The model under review builds one solid part; all positions refer to its coordinate system, in mm. Coordinates: 2 decimals unless noted, no trailing zeros. Write each loop counter-clockwise with the first axis right and the second up, starting at its lowest first coordinate (ties: lowest second). Pieces come first, ordered by that corner, then holes.
```python
from build123d import *

# Parameters (mm, degrees)
BOSS_EXTRUDE1_DEPTH  = 0.79375
M4_CLEARANCE_HOLE1_D = 4.8


with BuildPart() as part:
    # Sketch1 → Boss-Extrude1 (new, symmetric)
    with BuildSketch(Plane(origin=(0, 0, 0), x_dir=(0, 0, -1), z_dir=(1, 0, 0))):
        with BuildLine():
            Line((-5.08, 12.7), (-5.08, -6.538207725))
            ThreePointArc((-5.08, -6.538207725), (-5.211700121, -7.824771606), (-5.601337517, -9.057968362))
            Line((-5.601337517, -9.057968362), (-21.415741229, -45.63954689))
            ThreePointArc((-21.415741229, -45.63954689), (-7.844956242, -39.930269315), (2.000109042, -50.877266399))
            Line((2.000109042, -50.877266399), (5.062707082, -9.46401976))
            ThreePointArc((5.062707082, -9.46401976), (5.075675298, -9.230020736), (5.08, -8.995702545))
            Line((5.08, -8.995702545), (5.08, 12.7))
            ThreePointArc((5.08, 12.7), (0, 17.78), (-5.08, 12.7))
        make_face()
    extrude(amount=BOSS_EXTRUDE1_DEPTH, both=True)

    # M4 Clearance Hole1 (through all)
    with Locations(Plane(origin=(0.79375, 0, 0), x_dir=(0, 0, -1), z_dir=(1, 0, 0))):
        with Locations((0, 0), (0, 12.7), (0, -12.7)):
            Hole(M4_CLEARANCE_HOLE1_D / 2)


solid = part.part
```
Item 1: Take a section at D-D, the plane y = -12.7. Write out the cut boundary in (x, z).
Solved:
outline: (-0.79, -4.82) - (0.79, -4.82) - (0.79, -2.4) - (-0.79, -2.4) - close; (-0.79, 2.4) - (0.79, 2.4) - (0.79, 7.18) - (-0.79, 7.18) - close
Item 2: Mouldability with a two-part tool opening along Z and no side actions: class faces 1 (the face through (-0.794, -16, 2)), 2 (the face through (0, 3, 5.08)), 3 (the face through (0, 2, -5.08)), 4 (the face through (-0.011, 14.724, 1.29)) as pulls with the +Z half, pulls with the -Z half, needs draft (parallel to the pull), parting line crosses it, or undercut.
Solved:
face 1: needs draft
face 2: pulls with the +Z half
face 3: pulls with the -Z half
face 4: undercut
Item 3: For pin 1 (6 mm diameter, centred on y = -12.7, z = 0, fed in from -X); pin 2 (0.5 mm diameter, centred on x = 0, y = 6.5, fed in from +Z), all flat-tipped, find the tip position at first contact; note any pin that passes through.
Solved:
pin 1: stops at x = -0.79
pin 2: stops at z = 5.08
Item 4: Take a section at A-A, the plane x = 0.25. Write out the cut boundary in (y, z).
Solved:
outline: (-50.88, -2) - (-9.46, -5.06) arc R6.35 ccw to (-9, -5.08) - (12.7, -5.08) arc R5.08 ccw to (12.7, 5.08) - (-6.54, 5.08) arc R6.35 cw to (-9.06, 5.6) - (-45.64, 21.42) arc R12.7 cw to start; hole circle Ø4.8 at (-12.7, 0); hole circle Ø4.8 at (0, 0); hole circle Ø4.8 at (12.7, 0)
Item 5: Take a section at B-B, the plane y = 0. Write out the cut boundary in (x, z).
Solved:
outline: (-0.79, -5.08) - (0.79, -5.08) - (0.79, -2.4) - (-0.79, -2.4) - close; (-0.79, 2.4) - (0.79, 2.4) - (0.79, 5.08) - (-0.79, 5.08) - close
Item 6: To check wall thickness, follow line 1 along Y through (x, z) = (0.45, 0); line 2 along Z through (x, y) = (0.4, 6.5); line 3 along Y through (x, z) = (0.1, 1.5). State the ranges of each line that lie inside material, in increasing order.
Solved:
line 1: y = -45.36 to -15.1, -10.3 to -2.4, 2.4 to 10.3, 15.1 to 17.78
line 2: z = -5.08 to 5.08
line 3: y = -43.48 to -14.57, -10.83 to -1.87, 1.87 to 10.83, 14.57 to 17.55
Item 7: Take a section at C-C, the plane z = 0. Write out the cut boundary in (x, y).
Solved:
outline: (-0.79, -45.36) - (0.79, -45.36) - (0.79, -15.1) - (-0.79, -15.1) - close; (-0.79, -10.3) - (0.79, -10.3) - (0.79, -2.4) - (-0.79, -2.4) - close; (-0.79, 2.4) - (0.79, 2.4) - (0.79, 10.3) - (-0.79, 10.3) - close; (-0.79, 15.1) - (0.79, 15.1) - (0.79, 17.78) - (-0.79, 17.78) - close
